from build123d import *

# Parameters (mm, degrees)
SKETCH1_W                = 88.3412
SKETCH1_H                = 120.8024
BOSS_EXTRUDE1_DEPTH      = 5.7912
SKETCH6_R                = 1.4224
SKETCH6_R_2              = 1.497641053
CUT_EXTRUDE5_DEPTH       = 76.052547347
SKETCH7_W                = 29.367351422
SKETCH7_H                = 13.544863044
CUT_EXTRUDE6_DEPTH       = 76.052547347
CAVITY1_START            = -60.4012
CAVITY1_OUTLINE_W        = 5.7912
CAVITY1_OUTLINE_H        = 5.7912
CAVITY1_DEPTH            = 40.267466667
CAVITY1_START_2          = 20.133733333
CAVITY1_2_OUTLINE_W      = 5.7912
CAVITY1_2_OUTLINE_H      = 5.7912
CAVITY1_2_DEPTH          = 40.267466667
CAVITY1_3_OUTLINE_W      = 21.725466667
CAVITY1_3_OUTLINE_H      = 5.7912
CAVITY1_3_OUTLINE_W_2    = 27.516666667
CAVITY1_3_DEPTH          = 5.7912
CAVITY1_START_3          = 54.61
CAVITY1_4_OUTLINE_W      = 21.725466667
CAVITY1_4_OUTLINE_H      = 5.7912
CAVITY1_4_OUTLINE_W_2    = 27.516666667
CAVITY1_4_DEPTH          = 5.7912
CUT_EXTRUDE13_DEPTH      = 22.352
CUT_EXTRUDE13_DEPTH_BACK = 32.512
SKETCH8_R                = 1.27
SKETCH9_W                = 13.671222204
SKETCH9_H                = 3.060294153
CUT_EXTRUDE14_DEPTH      = 76.052547347


# Read off the part's stored shape, not the designer's step: Cavity1
with BuildPart() as part:
    # Sketch1 → Boss-Extrude1 (new body)
    with BuildSketch(Plane.XY):
        Rectangle(SKETCH1_W, SKETCH1_H)
    extrude(amount=BOSS_EXTRUDE1_DEPTH)

    # Sketch6 → Cut-Extrude5 (cut, through all)
    with BuildSketch(Plane.XY.offset(5.7912)):
        with Locations((0.2032, -22.564194219)):
            Circle(SKETCH6_R)
        with Locations((24.423695828, -19.744653869)):
            Circle(SKETCH6_R)
        with Locations((-1.949450117, 4.630928051)):
            Circle(SKETCH6_R_2)
        with Locations((27.953664088, 6.598815085)):
            Circle(SKETCH6_R)
    extrude(amount=-CUT_EXTRUDE5_DEPTH, mode=Mode.SUBTRACT)

    # Sketch7 → Cut-Extrude6 (cut, through all)
    with BuildSketch(Plane(origin=(0, 0, 0), x_dir=(-1, 0, 0), z_dir=(0, 0, -1))):
        with Locations((-20.155118324, -5.666932702)):
            Rectangle(SKETCH7_W, SKETCH7_H)
    extrude(amount=-CUT_EXTRUDE6_DEPTH, mode=Mode.SUBTRACT)

    # Cavity1 outline → Cavity1 (cut)
    with BuildSketch(Plane(origin=(0, 0, 0), x_dir=(1, 0, 0), z_dir=(0, 1, 0)).offset(CAVITY1_START)):
        with Locations((41.275, -2.8956)):
            Rectangle(CAVITY1_OUTLINE_W, CAVITY1_OUTLINE_H)
        with Locations((-41.275, -2.8956)):
            Rectangle(CAVITY1_OUTLINE_W, CAVITY1_OUTLINE_H)
    extrude(amount=CAVITY1_DEPTH, mode=Mode.SUBTRACT)

    # Cavity1 2 outline → Cavity1 2 (cut)
    with BuildSketch(Plane(origin=(0, 0, 0), x_dir=(1, 0, 0), z_dir=(0, 1, 0)).offset(CAVITY1_START_2)):
        with Locations((41.275, -2.8956)):
            Rectangle(CAVITY1_2_OUTLINE_W, CAVITY1_2_OUTLINE_H)
        with Locations((-41.275, -2.8956)):
            Rectangle(CAVITY1_2_OUTLINE_W, CAVITY1_2_OUTLINE_H)
    extrude(amount=CAVITY1_2_DEPTH, mode=Mode.SUBTRACT)

    # Cavity1 3 outline → Cavity1 3 (cut)
    with BuildSketch(Plane(origin=(0, 0, 0), x_dir=(1, 0, 0), z_dir=(0, 1, 0)).offset(CAVITY1_START)):
        with Locations((27.516666667, -2.8956)):
            Rectangle(CAVITY1_3_OUTLINE_W, CAVITY1_3_OUTLINE_H)
        with Locations((-24.621066667, -2.8956)):
            Rectangle(CAVITY1_3_OUTLINE_W_2, CAVITY1_3_OUTLINE_H)
    extrude(amount=CAVITY1_3_DEPTH, mode=Mode.SUBTRACT)

    # Cavity1 4 outline → Cavity1 4 (cut)
    with BuildSketch(Plane(origin=(0, 0, 0), x_dir=(1, 0, 0), z_dir=(0, 1, 0)).offset(CAVITY1_START_3)):
        with Locations((27.516666667, -2.8956)):
            Rectangle(CAVITY1_4_OUTLINE_W, CAVITY1_4_OUTLINE_H)
        with Locations((-24.621066667, -2.8956)):
            Rectangle(CAVITY1_4_OUTLINE_W_2, CAVITY1_4_OUTLINE_H)
    extrude(amount=CAVITY1_4_DEPTH, mode=Mode.SUBTRACT)

    # Sketch8 → Cut-Extrude13 (cut, two sides: drawn at the far end of the back side and taken through both)
    with BuildSketch(Plane.XY.offset(-CUT_EXTRUDE13_DEPTH_BACK)):
        with Locations(Location((-24.91218753, -46.860591388, 0), (0, 0, 180))):
            Circle(SKETCH8_R)
        with Locations(Location((-32.009882617, -39.878782893, 0), (0, 0, 180))):
            Circle(SKETCH8_R)
    extrude(amount=CUT_EXTRUDE13_DEPTH + CUT_EXTRUDE13_DEPTH_BACK, mode=Mode.SUBTRACT)

    # Sketch9 → Cut-Extrude14 (cut, through all)
    with BuildSketch(Plane.XY.offset(5.7912)):
        with Locations((-19.603898062, 35.76912754)):
            Rectangle(SKETCH9_W, SKETCH9_H)
    extrude(amount=-CUT_EXTRUDE14_DEPTH, mode=Mode.SUBTRACT)


solid = part.part
Verification items for the finished model (mm, model axes). A direction names the side the tool comes from. Coordinates: 2 decimals unless noted, no trailing zeros. Order: outer loops, then holes, each group sorted by start corner. A loop starts at its lowest first (then second) coordinate and runs counter-clockwise, first axis right, second up. Notation, with made-up numbers: M 29.25,25 L 57.25,25 A19 cw 57.25,46 Z; hole C 87,-9 d4. An arc over 180 degrees is marked long. Write each question's results on one line, items separated by ' | '.
1) Section check D-D on y = -51. Record the cut outline in (x, z).
Solved:
outline: M -38.38,0 L 38.38,0 L 38.38,5.79 L -38.38,5.79 Z
2) Section check A-A on x = 14. Record the cut outline in (y, z), plus the area to 3 significant figures.
Solved:
outline: M -60.4,0 L -12.44,0 L -12.44,5.79 L -60.4,5.79 Z; M 1.11,0 L 60.4,0 L 60.4,5.79 L 1.11,5.79 Z | area: 621 mm²
3) Access from +Z, -Z, +X, -X, +Y, -Y to the whole of each face (thin tool, end or side, straight path). Record for faces 1 (the face through (-25, 54.61, 3)), 2 (the face through (34.839, -6, 3)), 3 (the face through (38.379, -38, 3)), 4 (the face through (41, 20.134, 3)).
Solved:
face 1: +Z, -Z, -X, +Y | face 2: +Z, -Z | face 3: +Z, -Z, +X, -Y | face 4: +Z, -Z, +X, +Y
4) Gauge pin test, flat ends, axial feed: pin 1 Ø1.7 at (x, z) = (28, 2.5) entering from +Y; pin 2 Ø3 at (y, z) = (-33, 4.5) entering from -X; pin 3 Ø1.7 at (x, z) = (28, 3) entering from -Y. Record the tip position at first contact, or that the pin passes through.
Solved:
pin 1: stops at y = 54.61 | pin 2: stops at x = -38.38 | pin 3: stops at y = -54.61
5) Section check C-C on z = 2.85. Give the number of separate pieces and of enclosed holes in the cut face, plus the area to 3 significant figures.
Solved:
separate pieces: 1 | enclosed holes: 8 | area: 8,690 mm²
6) Release check for a two-part mould opening along X. For faces 5 (the face through (25.188, -18.545, 2.936)), 6 (the face through (20, -12.439, 3)), 7 (the face through (16.654, 57, 3)), 8 (the face through (-41, -20.134, 3)) record: pulls with the +X half, pulls with the -X half, needs draft (parallel to the pull), parting line crosses it, or undercut.
Solved:
face 5: undercut | face 6: undercut | face 7: pulls with the +X half | face 8: needs draft
7) Section check B-B on y = -7.5. Record the cut outline in (x, z), plus the area to 3 significant figures.
Solved:
outline: M -44.17,0 L 5.47,0 L 5.47,5.79 L -44.17,5.79 Z; M 34.84,0 L 44.17,0 L 44.17,5.79 L 34.84,5.79 Z | area: 342 mm²
8) Scan lines: line 1 along Y through (x, z) = (6, 5.45); line 2 along Y through (x, z) = (27, 0.4); line 3 along X through (y, z) = (-40, 0.8). Record each from-to range of solid material in increasing order. Write a range as [from, to].
Solved:
line 1: y = [-60.4, -12.44], [1.11, 60.4] | line 2: y = [-54.61, -12.44], [1.11, 5.54], [7.65, 54.61] | line 3: x = [-38.38, -33.27], [-30.75, 38.38]
